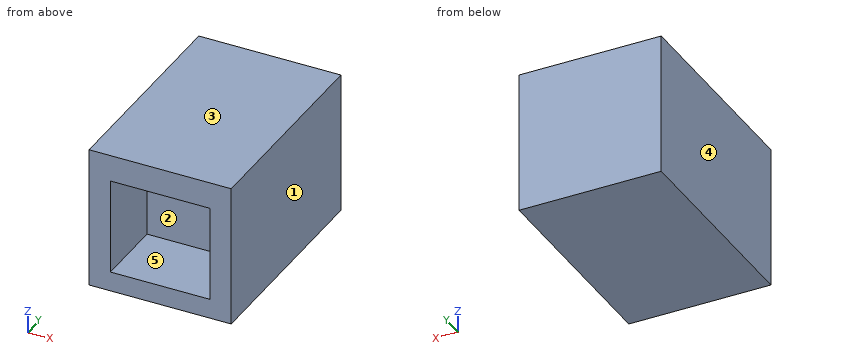
from build123d import *

# Parameters (mm, degrees)
F0_W      = 50.8
F0_H      = 50.8
F1_DEPTH  = 50.8
F1_FACE_W = 50.8
F1_FACE_H = 50.8
F2_DEPTH  = 25.4
F3_W      = 35.606458
F3_H      = 34.19029
F4_DEPTH  = 25.4


with BuildPart() as f1:
    # F0 (on Front) → F1 (new body)
    with BuildSketch(Plane.XZ):
        with Locations((-25.4, 25.4)):
            Rectangle(F0_W, F0_H)
    extrude(amount=F1_DEPTH)

    # F1_face (on face) → F2 (join)
    with BuildSketch(Plane(origin=(-25.4, -50.8, 25.4), x_dir=(1, 0, 0), z_dir=(0, -1, 0))):
        Rectangle(F1_FACE_W, F1_FACE_H)
    extrude(amount=F2_DEPTH)

    # F3 (on face) → F4 (cut)
    with BuildSketch(Plane.XZ.offset(76.2)):
        with Locations((-25.368032, 24.165593)):
            Rectangle(F3_W, F3_H)
    extrude(amount=-F4_DEPTH, mode=Mode.SUBTRACT)


solid = f1.part
Verification items for the finished model (mm, model axes). Face numbers are marked on the shaded views. A direction names the side the tool comes from. Coordinates: 2 decimals unless noted, no trailing zeros. Order: outer loops, then holes, each group sorted by start corner. A loop starts at its lowest first (then second) coordinate and runs counter-clockwise, first axis right, second up. Notation, with made-up numbers: (30.5, -33) -> (43.5, -33) arc R35 ccw to (43.5, 1) -> close; hole circle Ø1 at (40, 50.25). An arc over 180 degrees is marked (long way). Use CSV: the item, a comma, the result in double quotes. Start each with the question number.
Q1. Draft check along Z on the marked faces 3, 4 and 5. Enter one of: +Z half, -Z half, draft (parallel to the pull), parting line (faces both ways), or undercut.
Q2. Section check C-C, the plane z = 17. Record the cut outline in (x, y), and give its area (3 significant figures).
Q3. Thickness scan on line 1 along Z through (x, y) = (-15, -58.5); line 2 along X through (y, z) = (-72, 22); line 3 along Y through (x, z) = (-38.5, 23.5). Record the ranges inside material, lowest first.
Q4. Depth check by flat-ended pin: P1, Ø17, axis at x = -28, z = 29, coming from the -Y side. Enter the tip coordinate at first touch or a pass-through.
Q5. Section check A-A, the plane y = -66. Record the cut outline in (x, z).
Q6. Tool access check on the marked faces 1 and 2. Record the directions out of +Z, -Z, +X, -X, +Y, -Y that give a thin tool (end or side, any length) a straight path to the whole face; none if there is none.
Q7. Section check B-B, the plane x = -11. Record the cut outline in (y, z), and give its area (3 significant figures).
Returned:
1,face 3,"+Z half"
1,face 4,"draft"
1,face 5,"undercut"
2,outline,"(-50.8, -76.2) -> (-43.17, -76.2) -> (-43.17, -50.8) -> (-7.56, -50.8) -> (-7.56, -76.2) -> (0, -76.2) -> (0, 0) -> (-50.8, 0) -> close"
2,area,"2,970 mm^2"
3,line 1,"z = 0 to 7.07, 41.26 to 50.8"
3,line 2,"x = -50.8 to -43.17, -7.56 to 0"
3,line 3,"y = -50.8 to 0"
4,P1,"stops at y = -50.8"
5,outline,"(-50.8, 0) -> (0, 0) -> (0, 50.8) -> (-50.8, 50.8) -> close; hole (-43.17, 7.07) -> (-7.56, 7.07) -> (-7.56, 41.26) -> (-43.17, 41.26) -> close"
6,face 1,"+Z, -Z, +X, +Y, -Y"
6,face 2,"-Y"
7,outline,"(-76.2, 0) -> (0, 0) -> (0, 50.8) -> (-76.2, 50.8) -> (-76.2, 41.26) -> (-50.8, 41.26) -> (-50.8, 7.07) -> (-76.2, 7.07) -> close"
7,area,"3,000 mm^2"
